Geometry: final body of the model. Coordinates: model frame, mm. A direction names the side the tool comes from. Give positions to 0.01 mm unless a question says otherwise; leave off trailing zeros. Write each loop counter-clockwise with the first axis right and the second up, starting at its lowest first coordinate (ties: lowest second). Pieces come first, ordered by that corner, then holes. Notation, with made-up numbers: M 82,87.25 L 88,87.25 A14 ccw 88,95.25 Z; hole C 75,-3 d5. An arc over 180 degrees is marked long. One line per question, with ' | ' between items.
from build123d import *

# Parameters (mm, degrees)
SALIENTE_EXTRUIR1_DEPTH    = 12.5
CORTAR_EXTRUIR1_REACH      = 21.475
CROQUIS5_R                 = 2
CORTAR_EXTRUIR2_DEPTH      = 20.475369059
CORTAR_EXTRUIR2_DEPTH_BACK = 20.475369059


with BuildPart() as part:
    # Croquis4 → Saliente-Extruir1 (new, symmetric)
    with BuildSketch(Plane(origin=(0, 0, 0), x_dir=(0, 0, -1), z_dir=(1, 0, 0))):
        with BuildLine():
            Line((14, 0), (14, 0.7))
            Line((14, 0.7), (2.25, 0.7))
            ThreePointArc((2.25, 0.7), (1.5, 5.071320344), (3.664213562, 1.2))
            Line((3.664213562, 1.2), (4.624868417, 1.2))
            ThreePointArc((4.624868417, 1.2), (0.91958653, 5.582964109), (2.25, 0))
            Line((2.25, 0), (14, 0))
        make_face()
    extrude(amount=SALIENTE_EXTRUIR1_DEPTH, both=True)

    # Croquis5 → Cortar-Extruir1 (cut, up to next)
    with BuildSketch(Plane(origin=(0, 0.7, 0), x_dir=(1, 0, 0), z_dir=(0, 1, 0)), mode=Mode.PRIVATE) as cortar_extruir1_sk1:
        with Locations(Location((7, 8.5, 0), (0, 0, 270))):
            Circle(CROQUIS5_R)
    cortar_extruir1_tool1 = extrude(cortar_extruir1_sk1.sketch, amount=-CORTAR_EXTRUIR1_REACH, mode=Mode.PRIVATE) & part.part
    # Croquis5 → Cortar-Extruir1 (cut, up to next)
    with BuildSketch(Plane(origin=(0, 0.7, 0), x_dir=(1, 0, 0), z_dir=(0, 1, 0)), mode=Mode.PRIVATE) as cortar_extruir1_sk2:
        with Locations(Location((-7, 8.5, 0), (0, 0, 270))):
            Circle(CROQUIS5_R)
    cortar_extruir1_tool2 = extrude(cortar_extruir1_sk2.sketch, amount=-CORTAR_EXTRUIR1_REACH, mode=Mode.PRIVATE) & part.part
    add(cortar_extruir1_tool1.solids().sort_by_distance((7, 0.7, -8.5))[0], mode=Mode.SUBTRACT)
    add(cortar_extruir1_tool2.solids().sort_by_distance((-7, 0.7, -8.5))[0], mode=Mode.SUBTRACT)

    # Croquis6 → Cortar-Extruir2 (cut, two sides: drawn at the far end of the back side and taken through both)
    with BuildSketch(Plane(origin=(0, 0.7, 0), x_dir=(1, 0, 0), z_dir=(0, 1, 0)).offset(-CORTAR_EXTRUIR2_DEPTH_BACK)):
        Polygon((-5.75, 5.7), (-13.048594363, 5.7), (-13.048594363, -1.964735147), (14.193675093, -1.964735147), (14.193675093, 5.7), (5.75, 5.7), (5.75, -0.7), (-5.75, -0.7), align=None)
    extrude(amount=CORTAR_EXTRUIR2_DEPTH + CORTAR_EXTRUIR2_DEPTH_BACK, mode=Mode.SUBTRACT)


solid = part.part
(1) Set-up query: faces 4 (the face through (5.75, 1.4, -4.2)), 5 (the face through (8.352, 0.355, -9.974)), 6 (the face through (0, 0.7, -10)). Return all of +Z, -Z, +X, -X, +Y, -Y with unobstructed straight access to the full face (end or side cutting, diameter ignored); none if empty.
Working result:
face 4: +Z, +X, +Y, -Y | face 5: +Y, -Y | face 6: -Z, +X, -X
(2) Cut plane B-B, the plane z = -8.5. Return loops of the section in (x, y).
Working result:
outline: M -12.5,0 L -9,0 L -9,0.7 L -12.5,0.7 Z; M -5,0 L 5,0 L 5,0.7 L -5,0.7 Z; M 9,0 L 12.5,0 L 12.5,0.7 L 9,0.7 Z
(3) Cut plane A-A, the plane x = -7. Return loops of the section in (y, z), then the cut area to 3 significant figures.
Working result:
outline: M 0,-14 L 0.7,-14 L 0.7,-10.5 L 0,-10.5 Z; M 0,-6.5 L 0.7,-6.5 L 0.7,-5.7 L 0,-5.7 Z | area: 3.01 mm^2
(4) Draft query along X for faces 1 (the face through (-8.2, 0.4, -10.1)), 2 (the face through (0, 1.2, -4)), 3 (the face through (-5.75, 0.5, -2.5)). Return one class per face: released by +X, released by -X, zero draft, split by the parting line, or undercut.
Working result:
face 1: undercut | face 2: zero draft | face 3: released by -X
(5) First-contact query: P1, Ø1, axis at x = 2.5, y = 4.5, coming from the -Z side; P2, Ø2, axis at x = 3, y = 4, coming from the -Z side; P3, Ø1.8, axis at y = 4, z = -3.5, coming from the +X side. Flat tips, straight axial feed; report the tip coordinate or a pass-through.
Working result:
P1: stops at z = -5.01 | P2: stops at z = -5.2 | P3: stops at x = 5.75
(6) Material intervals for L1, parallel to X at y = 0.55, z = -8.5; L2, parallel to Z at x = -2.75, y = 2.95; L3, parallel to Y at x = 2.25, z = -4, sorted ascending. Write a range as [from, to].
Working result:
L1: x = [-12.5, -9], [-5, 5], [9, 12.5] | L2: z = [-5.2, -4.5], [0, 0.7] | L3: y = [0, 0.7], [1.2, 1.54], [4.36, 5.32]
(7) Cut plane D-D, the plane x = 2.25. Return loops of the section in (y, z).
Working result:
outline: M 0,-14 L 0.7,-14 L 0.7,-2.25 A2.25 cw long 1.2,-3.66 L 1.2,-4.62 A2.95 ccw long 0,-2.25 Z
(8) Cut plane C-C, the plane z = -0.25. Return loops of the section in (x, y).
Working result:
outline: M -5.75,0.78 L 5.75,0.78 L 5.75,1.92 L -5.75,1.92 Z; M -5.75,3.98 L 5.75,3.98 L 5.75,5.12 L -5.75,5.12 Z
